Verification items for the finished model (mm, model axes). Face numbers are marked on the shaded views. A direction names the side the tool comes from. Coordinates: 2 decimals unless noted, no trailing zeros. Write each loop counter-clockwise with the first axis right and the second up, starting at its lowest first coordinate (ties: lowest second). Pieces come first, ordered by that corner, then holes. Notation, with made-up numbers: (44, -13) - (81, -13) arc R34 ccw to (81, 23) - close; hole circle Ø6 at (-26, 37.5). An arc over 180 degrees is marked (long way). Use one line per item in the form item = value. Start each with the question number.
(1) Sectioned sample at D-D (z = 26). Record the cut outline in (x, y).
(2) Sectioned sample at B-B (y = -50). Record the cut outline in (x, z), and give its area (3 significant figures).
(3) Gauge pin test, flat ends, axial feed: pin 1 Ø1.5 at (x, z) = (-1.5, 10.5) entering from -Y; pin 2 Ø4 at (x, z) = (-2, 10.5) entering from -Y; pin 3 Ø1.5 at (x, z) = (7, 9) entering from +Y. Record the tip position at first contact, or that the pin passes through.
(4) Tool access check on the marked faces 4, 5 and 6. Record the directions out of +Z, -Z, +X, -X, +Y, -Y that give a thin tool (end or side, any length) a straight path to the whole face; none if there is none.
(5) Material ranges on line 1 (X direction, y = -50, z = 2); line 2 (Z direction, x = 10.5, y = -32); line 3 (Z direction, x = 12, y = -45), recorded low to high. Write a range as [from, to].
(6) Sectioned sample at A-A (x = 2). Record the cut outline in (y, z).
(7) Sectioned sample at C-C (z = 11). Record the cut outline in (x, y), and give its area (3 significant figures).
(8) Mould release check, pull along Y, two halves, no side actions. Record for the marked faces 1, 2 and 3: released by +Y, released by -Y, zero draft, split by the parting line, or undercut.
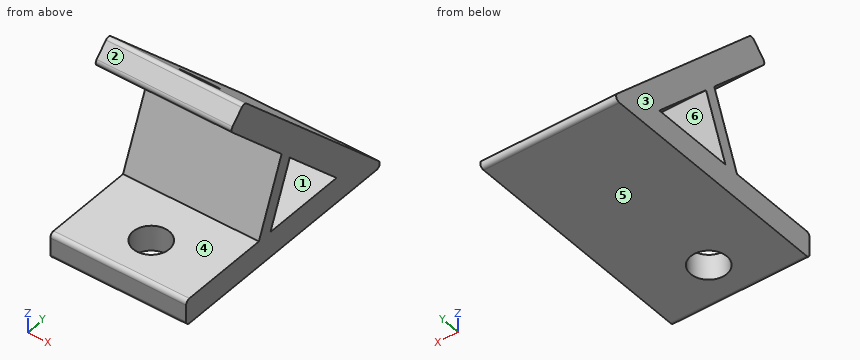
from build123d import *

# Parameters (mm, degrees)
PAD_DEPTH       = 16
SKETCH001_R     = 4.25
POCKET_DEPTH    = 6
SKETCH002_R     = 4.25
POCKET001_DEPTH = 6
FILLET_R        = 1


with BuildPart() as part:
    # Sketch → Pad (new body, symmetric)
    with BuildSketch(Plane.YZ):
        Polygon((-60, 0), (0, 0), (-42.4264068712, 42.4264068712), (-46.6690475583, 38.1837661841), (-31.1022907321, 22.6170093579), (-37.9852813742, 6), (-60, 6), align=None)
        Polygon((-28.627416998, 20.1421356237), (-34.4852813742, 6), (-14.4852813742, 6), align=None, mode=Mode.SUBTRACT)
    extrude(amount=PAD_DEPTH, both=True)

    # Sketch001 (on Face6 of Pad) → Pocket (cut)
    with BuildSketch(Plane(origin=(0, 0, 6), x_dir=(0, -1, 0), z_dir=(0, 0, 1))):
        with Locations((50, 0)):
            Circle(SKETCH001_R)
    extrude(amount=-POCKET_DEPTH, mode=Mode.SUBTRACT)

    # Sketch002 (on Face9 of Pocket) → Pocket001 (cut)
    with BuildSketch(Plane(origin=(0, -4.2426406871, -4.2426406871), x_dir=(0, 0.7071067812, -0.7071067812), z_dir=(0, -0.7071067812, -0.7071067812))):
        with Locations((-50, 0)):
            Circle(SKETCH002_R)
    extrude(amount=-POCKET001_DEPTH, mode=Mode.SUBTRACT)

    # Fillet
    fillet_edges = [part.edges().sort_by_distance(p)[0] for p in [
        (0, 0, 0),
        (0, -60, 0),
        (0, -60, 6),
        (0, -46.669048, 38.183766),
        (0, -42.426407, 42.426407),
    ]]
    fillet(fillet_edges, radius=FILLET_R)


solid = part.part
Answers below:
q1.outline = (-16, -34.49) - (16, -34.49) - (16, -26) - (-16, -26) - close
q2.outline = (-16, 0) - (-4.25, 0) - (-4.25, 6) - (-16, 6) - close; (4.25, 0) - (16, 0) - (16, 6) - (4.25, 6) - close
q2.area = 141 mm2
q3.pin_1 = -36.43
q3.pin_2 = -36.95
q3.pin_3 = -8.25
q4.face_4 = +X, -X, -Y
q4.face_5 = -Z, +X, -X, +Y, -Y
q4.face_6 = +X, -X
q5.line_1 = [-16, -4.25], [4.25, 16]
q5.line_2 = [0, 6], [12, 20.45], [23.51, 32]
q5.line_3 = [0, 6], [36.51, 39.85]
q6.outline = (-60, 1) arc R1 ccw to (-59, 0) - (-53.75, 0) - (-53.75, 6) - (-59, 6) arc R1 ccw to (-60, 5) - close; (-46.25, 0) - (-2.41, 0) arc R1 ccw to (-1.71, 1.71) - (-32.7, 32.7) - (-36.95, 28.46) - (-31.1, 22.62) - (-37.99, 6) - (-46.25, 6) - close; (-45.96, 37.48) - (-42.25, 33.76) - (-38.01, 38.01) - (-41.72, 41.72) arc R1 ccw to (-43.13, 41.72) - (-45.96, 38.89) arc R1 ccw to start; hole (-34.49, 6) - (-14.49, 6) - (-28.63, 20.14) - close
q7.outline = (-16, -35.91) - (16, -35.91) - (16, -32.41) - (-16, -32.41) - close; (-16, -19.49) - (16, -19.49) - (16, -11) - (-16, -11) - close
q7.area = 384 mm2
q8.face_1 = undercut
q8.face_2 = released by -Y
q8.face_3 = zero draft
